The listing builds one solid part. Answer for the finished solid, in the listing's coordinates (mm). Face numbers are marked on the shaded views. A direction names the side the tool comes from. Coordinates: 2 decimals unless noted, no trailing zeros. Loops run counter-clockwise (first coordinate to the right, second up) from the corner with the lowest first, then second, coordinate; pieces in that order, holes last. Notation, with made-up numbers: M -38.75,57.25 L 0.25,57.25 A21 ccw 0.25,86.25 Z; hole C -39.5,55.5 d8. An arc over 180 degrees is marked long. Return JSON: item names as keys, results as strings. Group by question number.
1. Straight lines are drawn through the part: L1, parallel to Y at x = 48, z = 1.35 (3 decimals); L2, parallel to Y at x = 27.5, z = 9.75 (3 decimals); L3, parallel to X at y = 12.75, z = 7.5. For each, find the intervals that lie inside material, in ascending order. Write a range as from..to.
2. Given P1, Ø1.5, axis at x = 24, y = 3, coming from the +Z side; P2, Ø4.5, axis at x = 7.5, y = 9.5, coming from the -Z side; P3, Ø0.5, axis at x = 17, z = 11, coming from the +Y side (3 decimals), each flat-ended and moving along its own axis, determine where each tip first touches the part or whether it passes through.
3. The mould has two halves that part along Y. Classify the marked faces 6, 7 and 8: pulls with the +Y half, pulls with the -Y half, needs draft (parallel to the pull), parting line crosses it, or undercut.
4. Section B-B (z = 7.25) is taken. Write down the section's boundary in (x, y) (3 decimals), then the cut area to 3 significant figures.
5. Which of the six approach directions +Z, -Z, +X, -X, +Y, -Y give full straight-line access (tool end or side, diameter ignored) to the marked faces 1, 2, 3, 4 and 5?
6. Section C-C (x = 48) is taken. Write down the section's boundary in (y, z) (3 decimals), then the cut area to 3 significant figures.
7. Section D-D (x = 34) is taken. Write down the section's boundary in (y, z).
8. Section A-A (x = 27.5) is taken. Write down the section's boundary in (y, z) (3 decimals).
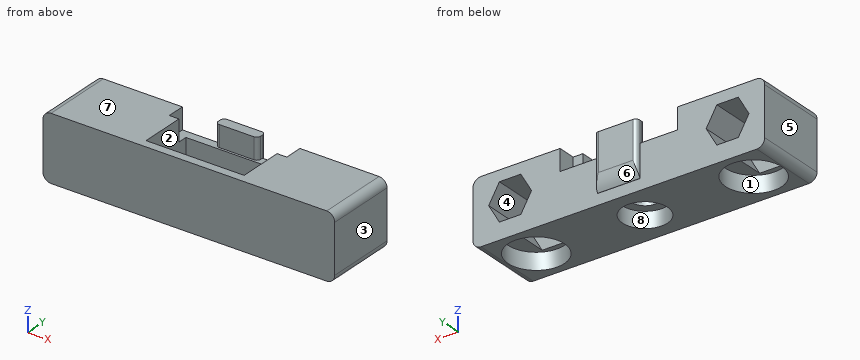
```python
from build123d import *

# Parameters (mm, degrees)
SKETCH2_W           = 55
SKETCH2_H           = 13.45
BOSS_EXTRUDE1_DEPTH = 12.2
SKETCH3_W           = 18.5
SKETCH3_H           = 10.25
CUT_EXTRUDE1_DEPTH  = 7.6
SKETCH5_W           = 22.15
SKETCH5_H           = 1.6
CUT_EXTRUDE2_DEPTH  = 4
SKETCH6_W           = 8
SKETCH6_H           = 2
BOSS_EXTRUDE2_DEPTH = 8.7
SKETCH7_W           = 1.825
SKETCH7_H           = 3.375
CUT_EXTRUDE3_DEPTH  = 4
FILLET1_R           = 0.75
FILLET3_R           = 0.75
DRAFT4_ANGLE        = 60
FILLET5_R           = 6
SKETCH8_R           = 2.5
CUT_EXTRUDE4_DEPTH  = 58.328314378
SKETCH9_R           = 4.25
CUT_EXTRUDE5_DEPTH  = 3
SKETCH10_R          = 5.3
CUT_EXTRUDE6_DEPTH  = 3.15
CUT_EXTRUDE7_DEPTH  = 11
FILLET6_R           = 1.5


with BuildPart() as part:
    # Sketch2 → Boss-Extrude1 (new body)
    with BuildSketch(Plane.XY):
        with Locations((27.5, 6.725)):
            Rectangle(SKETCH2_W, SKETCH2_H)
    extrude(amount=BOSS_EXTRUDE1_DEPTH)

    # Sketch3 → Cut-Extrude1 (cut)
    with BuildSketch(Plane.XY.offset(12.2)):
        with Locations((27.5, 6.725)):
            Rectangle(SKETCH3_W, SKETCH3_H)
    extrude(amount=-CUT_EXTRUDE1_DEPTH, mode=Mode.SUBTRACT)

    # Sketch5 → Cut-Extrude2 (cut)
    with BuildSketch(Plane.XY.offset(12.2)):
        with Locations((27.5, 12.65)):
            Rectangle(SKETCH5_W, SKETCH5_H)
    extrude(amount=-CUT_EXTRUDE2_DEPTH, mode=Mode.SUBTRACT)

    # Sketch6 → Boss-Extrude2 (add)
    with BuildSketch(Plane.XY.offset(12.2)):
        with Locations((27.5, 13.275)):
            Rectangle(SKETCH6_W, SKETCH6_H)
    extrude(amount=-BOSS_EXTRUDE2_DEPTH)

    # Sketch7 → Cut-Extrude3 (cut)
    with BuildSketch(Plane.XY.offset(12.2)):
        with Locations((37.6625, 11.7625)):
            Rectangle(SKETCH7_W, SKETCH7_H)
        with Locations((17.3375, 11.7625)):
            Rectangle(SKETCH7_W, SKETCH7_H)
    extrude(amount=-CUT_EXTRUDE3_DEPTH, mode=Mode.SUBTRACT)

    # Fillet1
    fillet1_edges = [part.edges().sort_by_distance(p)[0] for p in [
        (31.5, 14.275, 7.85),
        (31.5, 12.275, 10.2),
    ]]
    fillet(fillet1_edges, radius=FILLET1_R)

    # Fillet3
    fillet3_edges = [part.edges().sort_by_distance(p)[0] for p in [
        (23.5, 12.275, 10.2),
        (23.5, 14.275, 7.85),
    ]]
    fillet(fillet3_edges, radius=FILLET3_R)

    # Draft4
    draft4_faces = [part.faces().sort_by_distance(p)[0] for p in [
        (27.5, 13.853198642, 3.5),
    ]]
    draft(draft4_faces, Plane(origin=(23.5, 14.275, 3.5), x_dir=(0, 0, 1), z_dir=(0, 1, 0)), DRAFT4_ANGLE)

    # Fillet5
    # the kernel refuses this fillet: 6 mm, written as the material it takes off along each edge
    with BuildSketch(Plane(origin=(34.769237886, 14.275, 3.5), x_dir=(0, -0.49999999999999784, -0.8660254037844399), z_dir=(-1, 0, 0))) as fillet5_piece_1:
        with BuildLine():
            CenterArc((FILLET5_R * 0.267949192431, FILLET5_R), FILLET5_R, 240, 30)
            Line((-FILLET5_R * 0.232050807569, FILLET5_R * 0.133974596216), (0, 0))
            Line((0, 0), (FILLET5_R * 0.267949192431, 0))
        make_face()
    extrude(amount=14.538475773, mode=Mode.SUBTRACT)

    # Sketch8 → Cut-Extrude4 (cut, through all)
    with BuildSketch(Plane.XY.offset(4.6)):
        with Locations((27.5, 6.725)):
            Circle(SKETCH8_R)
    extrude(amount=-CUT_EXTRUDE4_DEPTH, mode=Mode.SUBTRACT)

    # Sketch9 → Cut-Extrude5 (cut)
    with BuildSketch(Plane(origin=(0, 0, 0), x_dir=(-1, 0, 0), z_dir=(0, 0, -1))):
        with Locations((-27.5, 6.725)):
            Circle(SKETCH9_R)
    extrude(amount=-CUT_EXTRUDE5_DEPTH, mode=Mode.SUBTRACT)

    # Sketch10 → Cut-Extrude6 (cut)
    with BuildSketch(Plane(origin=(0, 0, 0), x_dir=(-1, 0, 0), z_dir=(0, 0, -1))):
        with Locations((-48, 6.725)):
            Circle(SKETCH10_R)
        with Locations((-7, 6.725)):
            Circle(SKETCH10_R)
    extrude(amount=-CUT_EXTRUDE6_DEPTH, mode=Mode.SUBTRACT)

    # Sketch11 → Cut-Extrude7 (cut)
    with BuildSketch(Plane(origin=(0, 13.45, 0), x_dir=(1, 0, 0), z_dir=(0, 1, 0))):
        Polygon((9.020725942, -3.15), (4.979274058, -3.15), (2.958548116, -6.65), (4.979274058, -10.15), (9.020725942, -10.15), (11.041451884, -6.65), align=None)
        Polygon((43.958548116, -6.65), (45.979274058, -3.15), (50.020725942, -3.15), (52.041451884, -6.65), (50.020725942, -10.15), (45.979274058, -10.15), align=None)
    extrude(amount=-CUT_EXTRUDE7_DEPTH, mode=Mode.SUBTRACT)

    # Fillet6
    fillet6_edges = [part.edges().sort_by_distance(p)[0] for p in [
        (55, 6.725, 12.2),
        (0, 6.725, 12.2),
        (55, 6.725, 0),
        (0, 6.725, 0),
    ]]
    fillet(fillet6_edges, radius=FILLET6_R)


solid = part.part
```
Worked out:
{
 "1": {"L1": "0..1.425, 12.025..13.45", "L2": "0..1.6, 12.275..14.275", "L3": "0..3.45, 10.55..44.45, 51.55..55"},
 "2": {"P1": "z = 4.6", "P2": "z = 3.15", "P3": "y = 10.075"},
 "3": {"face 6": "pulls with the +Y half", "face 7": "needs draft", "face 8": "undercut"},
 "4": {"outline": "M 0,0 L 55,0 L 55,13.45 L 51.695,13.45 L 51.695,2.45 L 44.305,2.45 L 44.305,13.45 L 31.5,13.45 L 31.5,13.525 A0.75 ccw 30.75,14.275 L 24.25,14.275 A0.75 ccw 23.5,13.525 L 23.5,13.45 L 10.695,13.45 L 10.695,2.45 L 3.305,2.45 L 3.305,13.45 L 0,13.45 Z; hole M 18.25,1.6 L 36.75,1.6 L 36.75,11.85 L 18.25,11.85 Z", "area": "394 mm^2"},
 "5": {"face 1": "-Z", "face 2": "+Z", "face 3": "+Z, -Z, +X, +Y, -Y", "face 4": "+Y", "face 5": "+Z, -Z, -X, +Y, -Y"},
 "6": {"outline": "M 0,0 L 1.425,0 L 1.425,3.15 L 2.45,3.15 L 2.45,10.15 L 13.45,10.15 L 13.45,12.2 L 0,12.2 Z; M 12.025,0 L 13.45,0 L 13.45,3.15 L 12.025,3.15 Z", "area": "53.7 mm^2"},
 "7": {"outline": "M 0,0 L 13.45,0 L 13.45,8.2 L 11.85,8.2 L 11.85,4.6 L 1.6,4.6 L 1.6,12.2 L 0,12.2 Z"},
 "8": {"outline": "M 0,0 L 2.475,0 L 2.475,3 L 4.225,3 L 4.225,4.6 L 1.6,4.6 L 1.6,12.2 L 0,12.2 Z; M 9.225,3 L 10.975,3 L 10.975,0 L 13.45,0 L 13.45,2.071 L 13.471,2.108 A6 ccw 14.275,5.108 L 14.275,12.2 L 12.275,12.2 L 12.275,8.2 L 11.85,8.2 L 11.85,4.6 L 9.225,4.6 Z"}
}
